Source: CAD feature listing. Evaluate the final solid. Frame: model axes, mm. A direction names the side the tool comes from. Round coordinates to 2 decimals unless told otherwise and drop trailing zeros. Loops run counter-clockwise (first coordinate to the right, second up) from the corner with the lowest first, then second, coordinate; pieces in that order, holes last. Notation, with made-up numbers: M 76,41.5 L 134,41.5 A17 ccw 134,52.5 Z; hole C 78,41.5 d7. An arc over 180 degrees is marked long. Answer as a JSON object with one key per item and string values.
from build123d import *

# Parameters (mm, degrees)
SKETCH2_W           = 158.5
SKETCH2_H           = 195
BOSS_EXTRUDE1_DEPTH = 1.25
SKETCH1_W           = 156
SKETCH1_H           = 69.5
BOSS_EXTRUDE2_DEPTH = 105
SKETCH4_R           = 2.5
BOSS_EXTRUDE3_DEPTH = 8
FILLET2_R           = 2
SKETCH5_R           = 1.55
CUT_EXTRUDE1_DEPTH  = 8
SKETCH6_R           = 10
CUT_EXTRUDE2_DEPTH  = 8


with BuildPart() as part:
    # Sketch2 → Boss-Extrude1 (new body)
    with BuildSketch(Plane(origin=(0, 0, 0), x_dir=(1, 0, 0), z_dir=(0, 1, 0))):
        with Locations((0, -61.5)):
            Rectangle(SKETCH2_W, SKETCH2_H)
    extrude(amount=-BOSS_EXTRUDE1_DEPTH)

    # Sketch1 → Boss-Extrude2 (add)
    with BuildSketch(Plane(origin=(0, 0, 0), x_dir=(1, 0, 0), z_dir=(0, 1, 0))):
        Polygon((79.25, -159), (-79.25, -159), (-79.25, -86), (-79.25, -36), (-79.25, 36), (79.25, 36), (79.25, -36), (79.25, -86), align=None)
        Polygon((-78, -157.75), (78, -157.75), (78, -86), (78, -36), (-78, -36), (-78, -86), (-78, -100.588597569), align=None, mode=Mode.SUBTRACT)
        Rectangle(SKETCH1_W, SKETCH1_H, mode=Mode.SUBTRACT)
    extrude(amount=BOSS_EXTRUDE2_DEPTH)

    # Sketch4 → Boss-Extrude3 (add)
    with BuildSketch(Plane(origin=(0, 0, 0), x_dir=(1, 0, 0), z_dir=(0, 1, 0))):
        with Locations(Location((-37.075, -117.75, 0), (0, 0, 90))):
            Circle(SKETCH4_R)
        with Locations(Location((37.075, -117.75, 0), (0, 0, 90))):
            Circle(SKETCH4_R)
    extrude(amount=BOSS_EXTRUDE3_DEPTH)

    # Fillet2
    fillet2_edges = [part.edges().sort_by_distance(p)[0] for p in [
        (78, 52.5, -34.75),
        (78, 52.5, 34.75),
        (-78, 0, 0),
        (-78, 52.5, 34.75),
        (78, 52.5, 157.75),
        (-78, 52.5, 157.75),
        (0, 0, 36),
        (-78, 52.5, 36),
        (78, 0, 96.875),
        (78, 52.5, 36),
        (0, 0, -34.75),
        (-78, 52.5, -34.75),
        (0, 0, 157.75),
        (-78, 0, 96.875),
        (78, 0, 0),
        (0, 0, 34.75),
        (-37.075, 0, 120.25),
        (37.075, 0, 120.25),
    ]]
    fillet(fillet2_edges, radius=FILLET2_R)

    # Sketch5 → Cut-Extrude1 (cut)
    with BuildSketch(Plane.XY.offset(36)):
        with BuildLine():
            ThreePointArc((-53.75, 99.55), (-54.846015511, 99.096015511), (-55.3, 98))
            Line((-55.3, 98), (-53.75, 98))
            Line((-53.75, 98), (-53.75, 99.55))
        make_face()
        with BuildLine():
            Line((-53.75, 98), (-55.3, 98))
            ThreePointArc((-55.3, 98), (-53.75, 96.45), (-52.2, 98))
            ThreePointArc((-52.2, 98), (-52.653984489, 99.096015511), (-53.75, 99.55))
            Line((-53.75, 99.55), (-53.75, 98))
        make_face()
        with Locations((53.75, 98)):
            Circle(SKETCH5_R)
        with Locations((-53.75, 8)):
            Circle(SKETCH5_R)
        with Locations((53.75, 8)):
            Circle(SKETCH5_R)
    extrude(amount=-CUT_EXTRUDE1_DEPTH, mode=Mode.SUBTRACT)

    # Sketch6 → Cut-Extrude2 (cut)
    with BuildSketch(Plane(origin=(0, 0, 157.75), x_dir=(-1, 0, 0), z_dir=(0, 0, -1))):
        with Locations((0, 22)):
            Circle(SKETCH6_R)
    extrude(amount=-CUT_EXTRUDE2_DEPTH, mode=Mode.SUBTRACT)


solid = part.part
Item 1: Section B-B on z = 117.75. Return the cut outline in (x, y) (3 decimals).
Answer sheet:
{"outline": "M -79.25,-1.25 L 79.25,-1.25 L 79.25,105 L 78,105 L 78,2 A2 cw 76,0 L 41.575,0 A2 cw 39.575,2 L 39.575,8 L 34.575,8 L 34.575,2 A2 cw 32.575,0 L -32.575,0 A2 cw -34.575,2 L -34.575,8 L -39.575,8 L -39.575,2 A2 cw -41.575,0 L -76,0 A2 cw -78,2 L -78,105 L -79.25,105 Z"}
Item 2: Pull-direction query (X, two-part tool) for faces 4 (the flat face through (79.25, 51, 63)), 5 (the flat face through (-1, 0, 96)), 6 (the flat face through (78, 53, 96)), 7 (the flat face through (-1, 51, -36)); classes: pulls with the +X half, pulls with the -X half, needs draft (parallel to the pull), parting line crosses it, or undercut.
Answer sheet:
{"face 4": "pulls with the +X half", "face 5": "undercut", "face 6": "undercut", "face 7": "needs draft"}
Item 3: Line query: probe 1 along Z at (x, y) = (-7.5, 44.5); probe 2 along Y at (x, z) = (53.75, 35.3); probe 3 along Y at (x, z) = (0, 158). Output: solid intervals per line, ascending. Write a range as from..to.
Answer sheet:
{"probe 1": "z = -36..-34.75, 34.75..36, 157.75..159", "probe 2": "y = -1.25..6.45, 9.55..96.45, 99.55..105", "probe 3": "y = -1.25..12, 32..105"}
Item 4: Access query for faces 1 (the flat face through (-79.25, 51, 60)), 2 (the flat face through (-37, 8, 118)), 3 (the cylindrical face through (1.302, 31.915, 158.366)). Directions: +Z, -Z, +X, -X, +Y, -Y. A direction counts if a zero-diameter tool reaches every point of the face in a straight line with its end or side. Return the directions, or none.
Answer sheet:
{"face 1": "+Z, -Z, -X, +Y, -Y", "face 2": "+Y", "face 3": "+Z"}
Item 5: Contact query for a flat-ended pin moving along its axis: pin 1 Ø2.5 at (x, z) = (37.5, 118.5) entering from +Y. Output: stop coordinate, or through.
Answer sheet:
{"pin 1": "stops at y = 8"}
Item 6: Section A-A on y = 76.5. Return the cut outline in (x, z), then the cut area to 3 significant figures.
Answer sheet:
{"outline": "M -79.25,-36 L 79.25,-36 L 79.25,159 L -79.25,159 Z; hole M -78,-32.75 A2 ccw -76,-34.75 L 76,-34.75 A2 ccw 78,-32.75 L 78,32.75 A2 ccw 76,34.75 L -76,34.75 A2 ccw -78,32.75 Z; hole M -78,38 A2 ccw -76,36 L 76,36 A2 ccw 78,38 L 78,155.75 A2 ccw 76,157.75 L -76,157.75 A2 ccw -78,155.75 Z", "area": "1,080 mm²"}
Item 7: Section C-C on x = 60. Return the cut outline in (y, z), then the cut area to 3 significant figures.
Answer sheet:
{"outline": "M -1.25,-36 L 105,-36 L 105,-34.75 L 2,-34.75 A2 cw 0,-32.75 L 0,32.75 A2 cw 2,34.75 L 105,34.75 L 105,36 L 2,36 A2 cw 0,38 L 0,155.75 A2 cw 2,157.75 L 105,157.75 L 105,159 L -1.25,159 Z", "area": "641 mm²"}
Item 8: Section D-D on x = 1. Return the cut outline in (y, z), then the cut area to 3 significant figures.
Answer sheet:
{"outline": "M -1.25,-36 L 105,-36 L 105,-34.75 L 2,-34.75 A2 cw 0,-32.75 L 0,32.75 A2 cw 2,34.75 L 105,34.75 L 105,36 L 2,36 A2 cw 0,38 L 0,155.75 A2 cw 2,157.75 L 12.05,157.75 L 12.05,159 L -1.25,159 Z; M 31.95,157.75 L 105,157.75 L 105,159 L 31.95,159 Z", "area": "616 mm²"}
